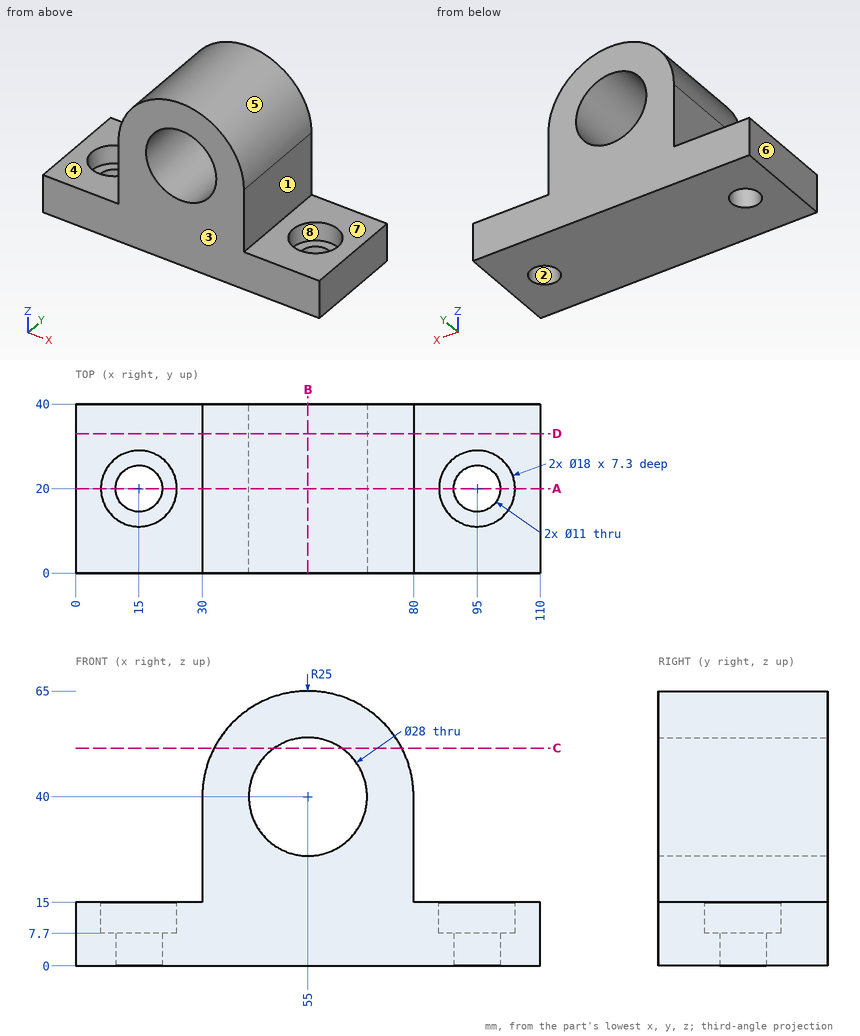
Can you work these out from the drawing? Everything is in mm from the part's minimum corner. A direction names the side the tool comes from. Round coordinates to 2 decimals unless told otherwise and drop trailing zeros. Order: outer loops, then holes, each group sorted by start corner. A loop starts at its lowest first (then second) coordinate and runs counter-clockwise, first axis right, second up.
(1) If we section it at D-D (y = 33): Please give me the cut outline in (x, z).
Results are:
outline: (0, 0) - (110, 0) - (110, 15) - (80, 15) - (80, 40) arc R25 ccw to (30, 40) - (30, 15) - (0, 15) - close; hole circle Ø28 at (55, 40)
(2) If I drill on L1, parallel to Z at x = 55, y = 13.5; L2, parallel to Y at x = 95, z = 10; L3, parallel to Y at x = 15, z = 3, over which ranges is the centre line in solid material (lowest first)?
Results are:
L1: z = 0 to 26, 54 to 65
L2: y = 0 to 11, 29 to 40
L3: y = 0 to 14.5, 25.5 to 40
(3) I'm going to push flat-ended pins straight in: pin 1 (6 mm diameter, centred on y = 22.5, z = 55, fed in from -X); pin 2 (2 mm diameter, centred on y = 17, z = 57, fed in from +X); pin 3 (1 mm diameter, centred on x = 65.5, y = 7, fed in from -Z); pin 4 (25 mm diameter, centred on x = 55, z = 40, fed in from +Y). Where does each tip first touch, or does it pass through?
Results are:
pin 1: stops at x = 33.07
pin 2: stops at x = 74.21
pin 3: stops at z = 0
pin 4: passes through
(4) If we section it at B-B (x = 55): Please give me the cut outline in (y, z).
Results are:
outline: (0, 0) - (40, 0) - (40, 26) - (0, 26) - close; (0, 54) - (40, 54) - (40, 65) - (0, 65) - close
(5) If we section it at C-C (z = 51.5): Please give me the cut outline in (x, y), plus the area to 3 significant figures.
Results are:
outline: (32.8, 0) - (47.02, 0) - (47.02, 40) - (32.8, 40) - close; (62.98, 0) - (77.2, 0) - (77.2, 40) - (62.98, 40) - close
area: 1,140 mm2
(6) We'd pull the mould along Y, two halves only. Please class the marked faces 1, 2 and 3: +Y half, -Y half, draft (parallel to the pull), parting line (faces both ways), or undercut.
Results are:
face 1: draft
face 2: undercut
face 3: -Y half
(7) If we section it at A-A (y = 20): Please give me the cut outline in (x, z).
Results are:
outline: (0, 0) - (9.5, 0) - (9.5, 7.7) - (6, 7.7) - (6, 15) - (0, 15) - close; (20.5, 0) - (89.5, 0) - (89.5, 7.7) - (86, 7.7) - (86, 15) - (80, 15) - (80, 40) arc R25 ccw to (30, 40) - (30, 15) - (24, 15) - (24, 7.7) - (20.5, 7.7) - close; (100.5, 0) - (110, 0) - (110, 15) - (104, 15) - (104, 7.7) - (100.5, 7.7) - close; hole circle Ø28 at (55, 40)
(8) On a 3-axis mill with a long thin cutter (end or side, diameter ignored), from which of +Z, -Z, +X, -X, +Y, -Y can I reach the whole of each face in a straight line? I mean the marked faces 4, 5, 6, 7 and 8. Say none if no direction works.
Results are:
face 4: +Z, -X, +Y, -Y
face 5: +Z, +Y, -Y
face 6: +Z, -Z, -X, +Y, -Y
face 7: +Z, +X, +Y, -Y
face 8: +Z
